Can you work these out from the model? Positions are in its coordinate system, mm. Face numbers are marked on the shaded views. A direction names the side the tool comes from. Round coordinates to 2 decimals unless told otherwise and drop trailing zeros. Order: outer loops, then holes, each group sorted by start corner. A loop starts at its lowest first (then second) coordinate and runs counter-clockwise, first axis right, second up.
from build123d import *

# Parameters (mm, degrees)
F0_W     = 105.22262
F0_H     = 32.062296
F1_DEPTH = 106.68
F0_W_2   = 106.097046
F0_H_2   = 53.922951
F2_DEPTH = 25.4
F3_DEPTH = 25.4


with BuildPart() as f1:
    # F0 (on Front) → F1 (new body)
    with BuildSketch(Plane.XZ):
        with Locations((-3.93492, -32.597718)):
            Rectangle(F0_W, F0_H)
    extrude(amount=F1_DEPTH)

    # F0 (on Front) → F2 (join)
    with BuildSketch(Plane.XZ):
        with Locations((-4.372133, 37.590868)):
            Rectangle(F0_W_2, F0_H_2)
        Polygon((48.67639, 10.629393), (-57.420656, 10.629393), (-56.54623, -16.56657), (48.67639, -16.56657), align=None)
        with Locations((-3.93492, -32.597718)):
            Rectangle(F0_W, F0_H)
    extrude(amount=F2_DEPTH)

    # F0 (on Front) → F3 (join)
    with BuildSketch(Plane.XZ):
        with Locations((-4.372133, 37.590868)):
            Rectangle(F0_W_2, F0_H_2)
        Polygon((48.67639, 10.629393), (-57.420656, 10.629393), (-56.54623, -16.56657), (48.67639, -16.56657), align=None)
        with Locations((-3.93492, -32.597718)):
            Rectangle(F0_W, F0_H)
    extrude(amount=F3_DEPTH)


solid = f1.part
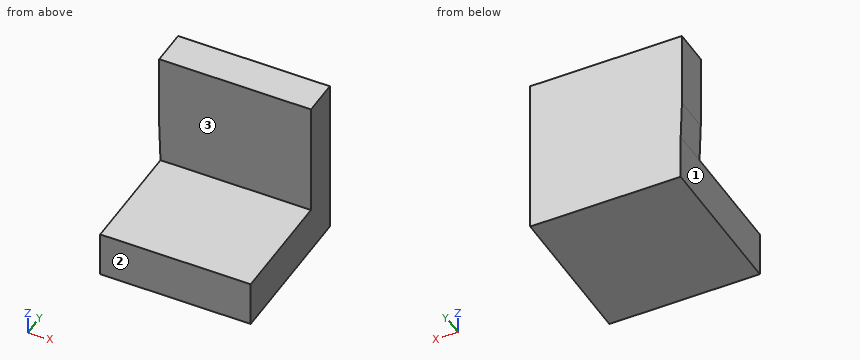
(1) Please list where these lines run through material, in increasing order: probe 1 along Z at (x, y) = (4.5, -66); probe 2 along Y at (x, z) = (-31, 35.5); probe 3 along X at (y, z) = (-24, -24).
(2) I'm going to push flat-ended pins straight in: pin 1 Ø1.5 at (x, z) = (33, 45) entering from -Y; pin 2 Ø3 at (x, y) = (19, -60) entering from +Z; pin 3 Ø9.5 at (y, z) = (-28.5, -40.5) entering from -X. Where does each tip first touch, or does it pass through?
(3) I want a section at A-A, the plane x = 5. List the corners of the cut face in (y, z) for me.
(4) I want a section at C-C, the plane z = 37. List the corners of the cut face in (x, y) for me, plus the area to 3 significant figures.
(5) On a 3-axis mill with a long thin cutter (end or side, diameter ignored), from which of +Z, -Z, +X, -X, +Y, -Y can I reach the whole of each face in a straight line? I mean the marked faces 1, 2 and 3. Say none if no direction works.
(6) I want a section at B-B, the plane y = -84. List the corners of the cut face in (x, z) for me.
Ans:
1. probe 1: z = -48.63 to -16.57
1. probe 2: y = -25.4 to 0
1. probe 3: x = -56.55 to 48.68
2. pin 1: stops at y = -25.4
2. pin 2: stops at z = -16.57
2. pin 3: stops at x = -56.55
3. outline: (-106.68, -48.63) - (0, -48.63) - (0, 64.55) - (-25.4, 64.55) - (-25.4, -16.57) - (-106.68, -16.57) - close
4. outline: (-57.42, -25.4) - (48.68, -25.4) - (48.68, 0) - (-57.42, 0) - close
4. area: 2,690 mm2
5. face 1: -Z, -X, +Y, -Y
5. face 2: +Z, -Z, +X, -X, -Y
5. face 3: +Z, +X, -X, -Y
6. outline: (-56.55, -48.63) - (48.68, -48.63) - (48.68, -16.57) - (-56.55, -16.57) - close
